from build123d import *

# Parameters (mm, degrees)
F2_SIZE = 2.54
F3_SIZE = 1.27


with BuildPart() as f1:
    # F0 (on Front) → F1 (revolve)
    with BuildSketch(Plane.XZ):
        Polygon((0, -228.6), (0, 228.6), (-25.4, 228.6), (-25.4, 0), (-20.2219, 0), (-20.2219, -12.7), (-11.674506, -38.1), (-14.372522, -38.1), (-14.372522, -190.5), (-11.674506, -190.5), (-11.674506, -196.85), (-18.241385, -196.85), (-18.241385, -203.2), align=None)
    revolve(axis=Axis((0, 0, 0), (0, 0, -1)))

    # F2
    f2_edges = [f1.edges().sort_by_distance(p)[0] for p in [
        (25.4, 0, 228.6),
    ]]
    chamfer(f2_edges, length=F2_SIZE)

    # F3
    f3_edges = [f1.edges().sort_by_distance(p)[0] for p in [
        (25.4, 0, 0),
        (14.372522, 0, -38.1),
        (18.241385, 0, -196.85),
        (14.372522, 0, -190.5),
    ]]
    chamfer(f3_edges, length=F3_SIZE)


solid = f1.part
Build history of the part. All positions in model axes, mm. A direction names the side the tool comes from. Round coordinates to 2 decimals unless told otherwise and drop trailing zeros. Order: outer loops, then holes, each group sorted by start corner. A loop starts at its lowest first (then second) coordinate and runs counter-clockwise, first axis right, second up. Notation, with made-up numbers: M 38,47 L 89,47 A12 cw 89,61 Z; hole C 72.25,69 d3. An arc over 180 degrees is marked long. Use CSV: the item, a comma, the result in double quotes. Start each with the question number.
(1) Flat gauge pins, fed straight in: P1, Ø10, axis at x = -15.5, y = -14, coming from the -Z side; P2, Ø4, axis at x = -19, z = -1, coming from the +Y side; P3, Ø14.5, axis at x = -0.5, y = 9, coming from the -Z side. Where does each tip first touch, or does it go through?
(2) Tool access for faces 5 (the face through (0, 0, 228.6)), 6 (the face through (-17.4, 5.48, -200.7)), 7 (the face through (-13.71, 4.32, -115.35)): list every direction of +Z, -Z, +X, -X, +Y, -Y with a clear straight run to the whole face (end or side of a thin tool).
(3) Mould opens along Z. For faces 1 (the face through (5.506, -24.796, 112.091)), 2 (the face through (3.92, -3.01, -221.72)), 3 (the face through (4, 12, -196.85)), 4 (the face through (-12.375, 19.41, 228.441)) say: +Z half, -Z half, draft (parallel to the pull), parting line (faces both ways), or undercut.
(4) Cut at B-B on z = -6. List the corners of the cut face in (x, y).
(5) Drill centre lines: probe 1 along Z at (x, y) = (10, -7); probe 2 along Y at (x, z) = (-1, -172); probe 3 along Z at (x, y) = (11.5, -13.5). Where is each one in solid material? Low to high.
(6) Cut at A-A on z = -147. List the corners of the cut face in (x, y), then the cut area to 3 significant figures.
Findings:
1,P1,"stops at z = -206.48"
1,P2,"stops at y = 17.17"
1,P3,"stops at z = -226.14"
2,face 5,"+Z, +X, -X, +Y, -Y"
2,face 6,"-Z"
2,face 7,"none"
3,face 1,"draft"
3,face 2,"-Z half"
3,face 3,"undercut"
3,face 4,"+Z half"
4,outline,"C 0,0 d40.44"
5,probe 1,"z = -211.6 to -196.85, -190.5 to -38.1, -36.52 to 228.6"
5,probe 2,"y = -14.34 to 14.34"
5,probe 3,"z = -203.91 to -197.61, -20.09 to 228.6"
6,outline,"C 0,0 d28.75"
6,area,"649 mm^2"
